Here's the drawing with two shaded views (mm, measured from the low corner). I have some questions. A direction names the side the tool comes from. Round coordinates to 2 decimals unless told otherwise and drop trailing zeros. Loops run counter-clockwise (first coordinate to the right, second up) from the corner with the lowest first, then second, coordinate; pieces in that order, holes last. Notation, with made-up numbers: M 26,37 L 67,37 A13 ccw 67,61 Z; hole C 79.5,-12.75 d10. An arc over 180 degrees is marked long. Answer as a JSON object with one key per item and string values.
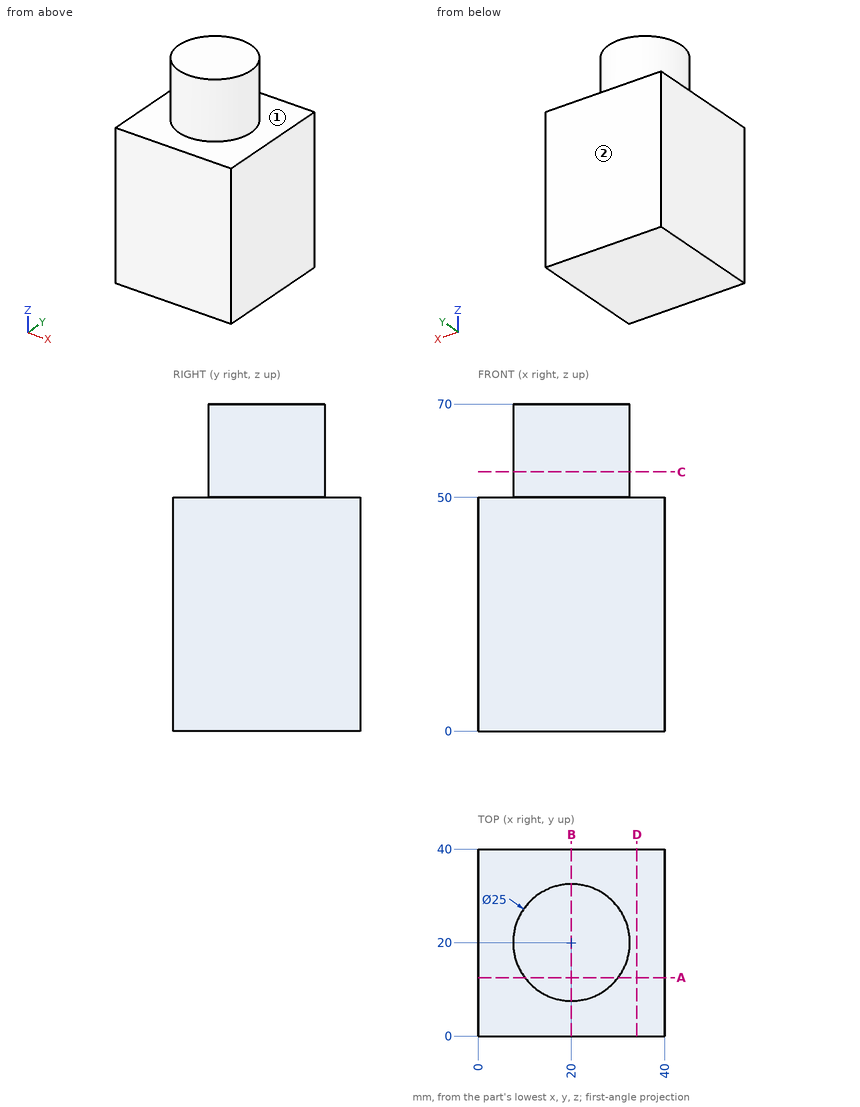
Item 1: For P1, Ø1.5, axis at x = 5.5, y = 34, coming from the +Z side; P2, Ø2, axis at y = 25, z = 59, coming from the -X side, each with a flat end and sliding along its axis, tell me the tip position at first contact or that it passes through.
Solution:
{"P1": "stops at z = 50", "P2": "stops at x = 8.16"}
Item 2: I want a section at D-D on x = 34. List the corners of the cut face in (y, z) for me.
Solution:
{"outline": "M 0,0 L 40,0 L 40,50 L 0,50 Z"}
Item 3: If I drill on L1, parallel to Z at x = 6, y = 28; L2, parallel to Y at x = 30.5, z = 51; L3, parallel to X at y = 13, z = 55, over which ranges is the centre line in solid material (lowest first)? Write a range as from..to.
Solution:
{"L1": "z = 0..50", "L2": "y = 13.22..26.78", "L3": "x = 9.64..30.36"}
Item 4: I want a section at C-C on z = 55.5. List the corners of the cut face in (x, y) for me.
Solution:
{"outline": "C 20,20 d25"}
Item 5: I want a section at A-A on y = 12.5. List the corners of the cut face in (x, z) for me, plus the area to 3 significant figures.
Solution:
{"outline": "M 0,0 L 40,0 L 40,50 L 30,50 L 30,70 L 10,70 L 10,50 L 0,50 Z", "area": "2,400 mm2"}
Item 6: I want a section at B-B on x = 20. List the corners of the cut face in (y, z) for me.
Solution:
{"outline": "M 0,0 L 40,0 L 40,50 L 32.5,50 L 32.5,70 L 7.5,70 L 7.5,50 L 0,50 Z"}
Item 7: For the marked faces 1 and 2, which set-ups out of +Z, -Z, +X, -X, +Y, -Y let a thin tool reach every point of the face, with its end or its side?
Solution:
{"face 1": "+Z", "face 2": "+Z, -Z, +X, -X, +Y"}
